from build123d import *

# Parameters (mm, degrees)
F1_DEPTH = 5


with BuildPart() as f1:
    # F0 (on Top) → F1 (new body)
    with BuildSketch(Plane.XY):
        with BuildLine():
            Line((0, 5), (-3, 5))
            ThreePointArc((-3, 5), (-3.912871, 4.408248), (-3.745356, 3.333333))
            Line((-3.745356, 3.333333), (-2.254644, 1.666667))
            ThreePointArc((-2.254644, 1.666667), (-2.087129, 0.591752), (-3, 0))
            Line((-3, 0), (0, 0))
            Line((0, 0), (0, 5))
        make_face()
    extrude(amount=F1_DEPTH)

    # F2: F1 across face


with BuildPart() as f1_1:
    add(f1.part)
    add(f1.part.mirror(Plane(origin=(0, 2.5, 2.5), x_dir=(0, 1, 0), z_dir=(1, 0, 0))))


solid = f1_1.part
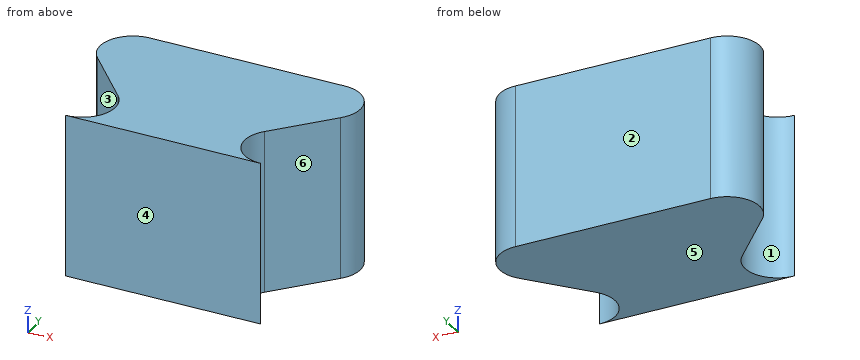
Design review of the part built by this model. Coordinates are the model's own, in mm. Face numbers are marked on the shaded views. A direction names the side the tool comes from. Coordinates: 2 decimals unless noted, no trailing zeros. Order: outer loops, then holes, each group sorted by start corner. A loop starts at its lowest first (then second) coordinate and runs counter-clockwise, first axis right, second up.
Item 1: For the marked faces 5 and 6, list the 3-axis set-ups (+Z, -Z, +X, -X, +Y, -Y) from which the entire face can be reached by the end or side of a thin tool; tool diameter is ignored.
Item 2: The part is to be moulded in two halves that separate along Y. For the marked faces 1, 2, 3 and 4, say which applies: pulls with the +Y half, pulls with the -Y half, needs draft (parallel to the pull), parting line crosses it, or undercut.
Item 3: For line 1 (X direction, y = 1.05, z = 2.2); line 2 (X direction, y = 3.05, z = 2); line 3 (Y direction, x = -3.25, z = 0.8), list the stretches that pass through material, from the lowest coordinate up.
Item 4: For pin 1 Ø1 at (y, z) = (2.5, 2.5) entering from +X, flat-tipped, find the tip position at first contact; note if it passes through.
Item 5: Take a section at B-B, the plane z = 2.65. Write out the cut boundary in (x, y), then the cut area to 3 significant figures.
Item 6: Take a section at D-D, the plane y = 2.6. Write out the cut boundary in (x, z).
Item 7: Take a section at C-C, the plane y = 1.4. Write out the cut boundary in (x, z).
The answers:
1. face 5: -Z, +X, -X, +Y, -Y
1. face 6: +Z, -Z, +X
2. face 1: undercut
2. face 2: pulls with the +Y half
2. face 3: undercut
2. face 4: pulls with the -Y half
3. line 1: x = -2 to 2
3. line 2: x = -3.49 to 3.49
3. line 3: y = 2.78 to 4.97
4. pin 1: stops at x = 3.45
5. outline: (-3.75, 3.33) - (-2.25, 1.67) arc R1 cw to (-3, 0) - (3, 0) arc R1 cw to (2.25, 1.67) - (3.75, 3.33) arc R1 ccw to (3, 5) - (-3, 5) arc R1 ccw to start
5. area: 30.0 mm2
6. outline: (-3.09, 0) - (3.09, 0) - (3.09, 5) - (-3.09, 5) - close
7. outline: (-2.08, 0) - (2.08, 0) - (2.08, 5) - (-2.08, 5) - close
